Could you check a few things on this model? Use its own coordinates, in mm. A direction names the side the tool comes from. Round coordinates to 2 decimals unless told otherwise and drop trailing zeros. Write each loop counter-clockwise with the first axis right and the second up, starting at its lowest first coordinate (ties: lowest second). Pieces come first, ordered by that corner, then holes. Notation, with made-up numbers: (25, 44.25) -> (69, 44.25) arc R33 ccw to (69, 83.25) -> close; hole circle Ø11 at (32.25, -13). An arc over 180 degrees is marked (long way). Answer as CSV lines item,"result". Start each with the question number.
Q1. Will these pins go through, and if not, where does the flat tip stop? pin 1 Ø5 at (x, z) = (-40.5, 21) entering from -Y; pin 2 Ø5.5 at (y, z) = (32.5, 20.5) entering from +X; pin 3 Ø2 at (x, y) = (-39.5, 95.5) entering from +Z.
Q2. If I drill on line 1 (X direction, y = 37, z = 33); line 2 (Y direction, x = -47, z = 17.5); line 3 (X direction, y = 82, z = -32), over which ranges is the centre line in solid material (lowest first)? Write a range as [from, to].
Q3. For faces 4 (the flat face through (-48.506, 132, 29)), 5 (the flat face through (-46.606, 101, -19)), 6 (the flat face through (-37, 184, 18)), 7 (the flat face through (-42, 15, -25.2)), 8 (the flat face through (-40, 105, 0)), which set-ups out of +Z, -Z, +X, -X, +Y, -Y let a thin tool reach every point of the face, with its end or its side?
Q4. If we mould it in two halves opening along Y, with no side actions, what happens to faces 1 (the flat face through (-39, 65, -22)), 2 (the flat face through (-38, 20, 18)), 3 (the flat face through (-42, 255.3, -15))? For each: pulls with the +Y half, pulls with the -Y half, needs draft (parallel to the pull), parting line crosses it, or undercut.
Q5. Imagine slicing it at D-D on z = -30.5. Please give me the cut outline in (x, y).
Q6. Imagine slicing it at B-B on z = 28.5. Please give me the cut outline in (x, y).
Q7. Imagine slicing it at A-A on y = 64.5. Please give me the cut outline in (x, z).
Q8. Imagine slicing it at C-C on y = 92.5. Please give me the cut outline in (x, z), and give its area (4 significant figures).
from build123d import *

# Parameters (mm, degrees)
BOSS_EXTRUDE1_DEPTH = 265.3
SKETCH2_W           = 10
SKETCH2_H           = 44
CUT_EXTRUDE1_DEPTH  = 10
SKETCH3_W           = 271.149403365
SKETCH3_H           = 159.03985052
CUT_EXTRUDE2_DEPTH  = 31
SKETCH4_W           = 28
SKETCH4_H           = 7
CUT_EXTRUDE3_DEPTH  = 8
SKETCH5_W           = 28.4
SKETCH5_H           = 7.4
CUT_EXTRUDE4_DEPTH  = 8
SKETCH6_W           = 44
SKETCH6_H           = 78
CUT_EXTRUDE5_DEPTH  = 18.3
SKETCH7_W           = 40
SKETCH7_H           = 51
CUT_EXTRUDE6_DEPTH  = 18.3
SKETCH8_W           = 3.9
SKETCH8_H           = 7
BOSS_EXTRUDE2_DEPTH = 44
CUT_EXTRUDE7_DEPTH  = 7
LPATTERN1_COUNT     = 2
LPATTERN1_PITCH     = 68
SKETCH11_W          = 4.5
SKETCH11_H          = 29.5
CUT_EXTRUDE8_DEPTH  = 15


with BuildPart() as part:
    # Sketch1 → Boss-Extrude1 (new body)
    with BuildSketch(Plane(origin=(0, 0, 0), x_dir=(1, 0, 0), z_dir=(0, 1, 0))):
        Polygon((-51.505795374, 37), (-32.205795374, 37), (-32.205795374, -18), (-42.205795374, -18), (-42.205795374, -37), (-45.205795374, -37), (-45.205795374, -22), (-48.505795374, -22), (-48.505795374, -37), (-51.505795374, -37), align=None)
    extrude(amount=BOSS_EXTRUDE1_DEPTH)

    # Sketch2 → Cut-Extrude1 (cut)
    with BuildSketch(Plane(origin=(0, 265.3, 0), x_dir=(1, 0, 0), z_dir=(0, 1, 0))):
        with Locations((-41.505795374, 15)):
            Rectangle(SKETCH2_W, SKETCH2_H)
    extrude(amount=-CUT_EXTRUDE1_DEPTH, mode=Mode.SUBTRACT)

    # Sketch3 → Cut-Extrude2 (cut)
    with BuildSketch(Plane(origin=(-25.752897687, 25.752897687, 0), x_dir=(0, 0, 1), z_dir=(0.7071067811865488, -0.7071067811865464, 0))):
        with Locations((3.075588753, 19.523863597)):
            Rectangle(SKETCH3_W, SKETCH3_H)
    extrude(amount=CUT_EXTRUDE2_DEPTH, mode=Mode.SUBTRACT)

    # Sketch4 → Cut-Extrude3 (cut)
    with BuildSketch(Plane(origin=(-25.752897687, 25.752897687, 0), x_dir=(0, 0, -1), z_dir=(0.7071067811865487, -0.7071067811865465, 0))):
        with Locations((11, -18.625775426)):
            Rectangle(SKETCH4_W, SKETCH4_H)
    extrude(amount=-CUT_EXTRUDE3_DEPTH, mode=Mode.SUBTRACT)

    # Sketch5 → Cut-Extrude4 (cut)
    with BuildSketch(Plane(origin=(-25.752897687, 25.752897687, 0), x_dir=(0, 0, -1), z_dir=(0.7071067811865487, -0.7071067811865465, 0))):
        with Locations((11, -18.625775426)):
            Rectangle(SKETCH5_W, SKETCH5_H)
    extrude(amount=-CUT_EXTRUDE4_DEPTH, mode=Mode.SUBTRACT)

    # Sketch6 → Cut-Extrude5 (cut)
    with BuildSketch(Plane(origin=(-32.205795374, 0, 0), x_dir=(0, 0, -1), z_dir=(1, 0, 0))):
        with Locations((0, 66)):
            Rectangle(SKETCH6_W, SKETCH6_H)
    extrude(amount=-CUT_EXTRUDE5_DEPTH, mode=Mode.SUBTRACT)

    # Sketch7 → Cut-Extrude6 (cut)
    with BuildSketch(Plane(origin=(-50.505795374, 0, 0), x_dir=(0, 0, -1), z_dir=(1, 0, 0))):
        with Locations((0, 70.5)):
            Rectangle(SKETCH7_W, SKETCH7_H)
    extrude(amount=-CUT_EXTRUDE6_DEPTH, mode=Mode.SUBTRACT)

    # Sketch8 → Boss-Extrude2 (add)
    with BuildSketch(Plane.XY.offset(-22)):
        with Locations((-48.555795374, 33.5)):
            Rectangle(SKETCH8_W, SKETCH8_H)
    boss_extrude2 = extrude(amount=BOSS_EXTRUDE2_DEPTH)

    # Sketch10 → Cut-Extrude7 (cut)
    with BuildSketch(Plane(origin=(0, 37, 0), x_dir=(1, 0, 0), z_dir=(0, 1, 0))):
        Polygon((-46.605795374, -15.29), (-48.505795374, -12.001413069), (-48.505795374, 11.998586931), (-46.605795374, 15.287173861), align=None)
    cut_extrude7 = extrude(amount=-CUT_EXTRUDE7_DEPTH, mode=Mode.SUBTRACT)

    # LPattern1: Boss-Extrude2, Cut-Extrude7 ×2
    with Locations(*[(0, i * LPATTERN1_PITCH, 0) for i in range(1, LPATTERN1_COUNT)]):
        add(boss_extrude2)
        add(cut_extrude7, mode=Mode.SUBTRACT)

    # Sketch11 → Cut-Extrude8 (cut)
    with BuildSketch(Plane.XY.offset(-22)):
        with Locations((-43.255795374, 75.25)):
            Rectangle(SKETCH11_W, SKETCH11_H)
    extrude(amount=-CUT_EXTRUDE8_DEPTH, mode=Mode.SUBTRACT)


solid = part.part
Checks:
1,pin 1,"y = 8.51"
1,pin 2,"x = -42.21"
1,pin 3,"z = -22"
2,line 1,"[-51.51, -48.51], [-45.21, -42.21]"
2,line 2,"[4.51, 27], [30, 37], [98, 265.3]"
2,line 3,"[-51.51, -45.51], [-41.01, -32.21]"
3,face 4,"+Z, +Y, -Y"
3,face 5,"+Z, +X"
3,face 6,"+Z, +X, +Y, -Y"
3,face 7,"none"
3,face 8,"+X"
4,face 1,"undercut"
4,face 2,"needs draft"
4,face 3,"pulls with the +Y half"
5,outline,"(-51.51, 0) -> (-32.21, 19.3) -> (-32.21, 265.3) -> (-36.51, 265.3) -> (-36.51, 255.3) -> (-46.51, 255.3) -> (-46.51, 265.3) -> (-51.51, 265.3) -> close; hole (-45.51, 60.5) -> (-41.01, 60.5) -> (-41.01, 90) -> (-45.51, 90) -> close"
6,outline,"(-51.51, 0) -> (-48.51, 3) -> (-48.51, 265.3) -> (-51.51, 265.3) -> close; (-45.21, 6.3) -> (-42.21, 9.3) -> (-42.21, 265.3) -> (-45.21, 265.3) -> close"
7,outline,"(-51.51, -37) -> (-45.51, -37) -> (-45.51, -22) -> (-50.51, -22) -> (-50.51, -20) -> (-51.51, -20) -> close; (-51.51, 20) -> (-50.51, 20) -> (-50.51, 22) -> (-48.51, 22) -> (-48.51, 37) -> (-51.51, 37) -> close; (-45.21, 22) -> (-42.21, 22) -> (-42.21, 37) -> (-45.21, 37) -> close; (-41.01, -37) -> (-32.21, -37) -> (-32.21, -22) -> (-41.01, -22) -> close"
8,outline,"(-51.51, -37) -> (-32.21, -37) -> (-32.21, -22) -> (-50.51, -22) -> (-50.51, -20) -> (-51.51, -20) -> close; (-51.51, 20) -> (-50.51, 20) -> (-50.51, 22) -> (-48.51, 22) -> (-48.51, 37) -> (-51.51, 37) -> close; (-45.21, 22) -> (-42.21, 22) -> (-42.21, 37) -> (-45.21, 37) -> close"
8,area,"383.5 mm^2"
